The listing builds one solid part. Answer for the finished solid, in the listing's coordinates (mm). A direction names the side the tool comes from. Coordinates: 2 decimals unless noted, no trailing zeros. Loops run counter-clockwise (first coordinate to the right, second up) from the corner with the lowest first, then second, coordinate; pieces in that order, holes last. Notation, with made-up numbers: (-5.5, -9) - (31.5, -9) arc R30 ccw to (31.5, 30) - close; hole circle Ø10 at (54.5, -16.5). An arc over 180 degrees is marked (long way). Put each result on its own line as item: value.
```python
from build123d import *

# Parameters (mm, degrees)
BOSS_EXTRUDE1_DEPTH         = 50.8
F_3_8_16_TAPPED_HOLE1_D     = 7.9375
F_3_8_16_TAPPED_HOLE1_DEPTH = 25.4
F_3_8_16_TAPPED_HOLE1_TIP   = 2.384665582
F_3_8_16_TAPPED_HOLE2_D     = 7.9375
F_3_8_16_TAPPED_HOLE2_DEPTH = 25.4
F_3_8_16_TAPPED_HOLE2_TIP   = 2.384665582


with BuildPart() as part:
    # Sketch1 → Boss-Extrude1 (new body)
    with BuildSketch(Plane.XY):
        Polygon((-76.2, 0), (76.2, 0), (76.2, 77.459343803), (-76.2, 25.4), align=None)
    extrude(amount=-BOSS_EXTRUDE1_DEPTH)

    # 3/8-16 Tapped Hole1
    with Locations(Plane(origin=(-15.732418717, 46.055528891, 0), x_dir=(0.946311265, 0.323256847, 0), z_dir=(-0.323256847, 0.946311265, 0))):
        with Locations((-38.143756412, 12.7), (71.393743588, 38.1)):
            Hole(F_3_8_16_TAPPED_HOLE1_D / 2, depth=F_3_8_16_TAPPED_HOLE1_DEPTH)
            with Locations((0, 0, -(F_3_8_16_TAPPED_HOLE1_DEPTH + F_3_8_16_TAPPED_HOLE1_TIP / 2))):  # 118° drill point
                Cone(0, F_3_8_16_TAPPED_HOLE1_D / 2, F_3_8_16_TAPPED_HOLE1_TIP, mode=Mode.SUBTRACT)

    # 3/8-16 Tapped Hole2
    with Locations(Plane(origin=(0, 0, 0), x_dir=(-1, 0, 0), z_dir=(0, -1, 0))):
        with Locations((38.1, 25.4), (-38.1, 25.4)):
            Hole(F_3_8_16_TAPPED_HOLE2_D / 2, depth=F_3_8_16_TAPPED_HOLE2_DEPTH)
            with Locations((0, 0, -(F_3_8_16_TAPPED_HOLE2_DEPTH + F_3_8_16_TAPPED_HOLE2_TIP / 2))):  # 118° drill point
                Cone(0, F_3_8_16_TAPPED_HOLE2_D / 2, F_3_8_16_TAPPED_HOLE2_TIP, mode=Mode.SUBTRACT)


solid = part.part
```
1) The part is cut by section A-A (z = -19). Give the vertices of the cut face in (x, y), and give its area (3 significant figures).
Found:
outline: (-76.2, 0) - (76.2, 0) - (76.2, 77.46) - (-76.2, 25.4) - close
area: 7,840 mm^2
2) The part is cut by section B-B (x = -3). Give the vertices of the cut face in (y, z), and give its area (3 significant figures).
Found:
outline: (0, -50.8) - (50.4, -50.8) - (50.4, 0) - (0, 0) - close
area: 2,560 mm^2
3) Each of these flat-tipped pins is pushed along its axis until it touches: pin 1 (6 mm diameter, centred on x = -3, z = -19.5, fed in from +Y); pin 2 (5 mm diameter, centred on x = -44, z = -8, fed in from +Y); pin 3 (12.5 mm diameter, centred on x = -38.1, z = -25.4, fed in from +Y); pin 4 (1 mm diameter, centred on x = 31.5, y = 11, fed in from +Z). Where does it stop, or does it pass through?
Found:
pin 1: stops at y = 51.43
pin 2: stops at y = 37.25
pin 3: stops at y = 40.55
pin 4: stops at z = 0
4) Straight lines are drawn through the part: L1, parallel to X at y = 18, z = -25.4; L2, parallel to X at y = 18, z = -25; L3, parallel to Z at x = 38.1, y = 14.75. For each, find the intervals that lie inside material, in ascending order. Write a range as [from, to].
Found:
L1: x = [-76.2, -42.07], [-34.13, 34.13], [42.07, 76.2]
L2: x = [-76.2, -42.05], [-34.15, 34.15], [42.05, 76.2]
L3: z = [-50.8, -29.37], [-21.43, 0]
5) For a pull along X with two mould halves and no side action, classify faces 4 (the face through (58.76, 57.89, -40.78)), 5 (the face through (16, 31, -50.8)), 6 (the face through (76.2, 38, -25)) as pulls with the +X half, pulls with the -X half, needs draft (parallel to the pull), parting line crosses it, or undercut.
Found:
face 4: undercut
face 5: needs draft
face 6: pulls with the +X half
6) For faces 1 (the face through (35.175, 12.878, -28.082)), 2 (the face through (60.02, 43.01, -38.13)), 3 (the face through (1.067, 51.794, -25.044)), determine the directions among +Z, -Z, +X, -X, +Y, -Y from which every point of the face is accessible in a straight line to the end or side of a thin tool.
Found:
face 1: -Y
face 2: none
face 3: +Z, -Z, -X, +Y
